```python
from build123d import *

# Parameters (mm, degrees)
SZKIC1_W                       = 168
SZKIC1_H                       = 88
ODGI_CIE_BAZOWE1_DEPTH         = 3
USKOK1_START                   = -44
USKOK1_DEPTH                   = 88
USKOK1_2_DEPTH                 = 88
SZKIC7_W                       = 60
SZKIC7_H                       = 40
WYTNIJ_WYCI_GNI_CIE1_DEPTH     = 113.751940116
ZAOKR_GLENIE1_R                = 5
OTWORY_USTALAJ_CE_6_2MM1_D     = 6.2
OTWORY_USTALAJ_CE_6_2MM1_DEPTH = 27.5
OTWORY_USTALAJ_CE_6_2MM1_TIP   = 1.862667919
OTWORY_USTALAJ_CE_8_0MM2_D     = 8.2
OTWORY_USTALAJ_CE_8_0MM2_DEPTH = 27.5
OTWORY_USTALAJ_CE_8_0MM2_TIP   = 2.463528538


# Read off the part's stored shape, not the designer's step: Uskok1
# Sheet-metal steps are written as plain solids
with BuildPart() as part:
    # Szkic1 → Odgięcie bazowe1 (new body)
    with BuildSketch(Plane(origin=(0, 0, 0), x_dir=(1, 0, 0), z_dir=(0, 1, 0))):
        Rectangle(SZKIC1_W, SZKIC1_H)
    extrude(amount=-ODGI_CIE_BAZOWE1_DEPTH)

    # Uskok1 outline → Uskok1 (cut)
    with BuildSketch(Plane.XY.offset(USKOK1_START)):
        with BuildLine():
            ThreePointArc((-10.756621532, 0), (-8.389154531, -0.845704021), (-7.093344311, -3))
            Line((-7.093344311, -3), (84, -3))
            Line((84, -3), (84, 0))
            Line((84, 0), (-10.756621532, 0))
        make_face()
    extrude(amount=USKOK1_DEPTH, mode=Mode.SUBTRACT)

    # Uskok1 2 outline → Uskok1 2 (add)
    with BuildSketch(Plane.XY.offset(USKOK1_START)):
        with BuildLine():
            ThreePointArc((-10.756621532, -3), (-10.235766677, -3.215745145), (-10.020021532, -3.7366))
            Line((-10.020021532, -3.7366), (-10.020021532, -60.2634))
            ThreePointArc((-10.020021532, -60.2634), (-8.925596731, -62.905575199), (-6.283421532, -64))
            Line((-6.283421532, -64), (84, -64))
            Line((84, -64), (84, -61))
            Line((84, -61), (-6.283421532, -61))
            ThreePointArc((-6.283421532, -61), (-6.804276387, -60.784254855), (-7.020021532, -60.2634))
            Line((-7.020021532, -60.2634), (-7.020021532, -3.7366))
            ThreePointArc((-7.020021532, -3.7366), (-7.038397411, -3.36647982), (-7.093344311, -3))
            Line((-7.093344311, -3), (-10.756621532, -3))
        make_face()
    extrude(amount=USKOK1_2_DEPTH)

    # Szkic7 → Wytnij-wyciągnięcie1 (cut, through all)
    with BuildSketch(Plane(origin=(0, -61, 0), x_dir=(1, 0, 0), z_dir=(0, 1, 0))):
        with Locations((54, 0)):
            Rectangle(SZKIC7_W, SZKIC7_H)
    extrude(amount=-WYTNIJ_WYCI_GNI_CIE1_DEPTH, mode=Mode.SUBTRACT)

    # Zaokrąglenie1
    zaokr_glenie1_edges = [part.edges().sort_by_distance(p)[0] for p in [
        (84, -62.5, -44),
        (84, -62.5, 44),
        (84, -62.5, -20),
        (84, -62.5, 20),
        (24, -62.5, 20),
        (24, -62.5, -20),
        (-84, -1.5, 44),
        (-84, -1.5, -44),
    ]]
    fillet(zaokr_glenie1_edges, radius=ZAOKR_GLENIE1_R)

    # Otwory ustalające Ø6.2mm1
    with Locations(Plane(origin=(0, -61, 0), x_dir=(1, 0, 0), z_dir=(0, 1, 0))):
        with Locations((74, 34.742873432), (74, -34.697126568), (4.56, -34.697126568), (4.56, 34.742873432)):
            Hole(OTWORY_USTALAJ_CE_6_2MM1_D / 2, depth=OTWORY_USTALAJ_CE_6_2MM1_DEPTH)
            with Locations((0, 0, -(OTWORY_USTALAJ_CE_6_2MM1_DEPTH + OTWORY_USTALAJ_CE_6_2MM1_TIP / 2))):  # 118° drill point
                Cone(0, OTWORY_USTALAJ_CE_6_2MM1_D / 2, OTWORY_USTALAJ_CE_6_2MM1_TIP, mode=Mode.SUBTRACT)

    # Otwory ustalające Ø8.0mm2
    with Locations(Plane(origin=(0, 0, 0), x_dir=(1, 0, 0), z_dir=(0, 1, 0))):
        with Locations((-69.878310766, 30), (-19.878310766, 30), (-19.878310766, -30), (-69.878310766, -30)):
            Hole(OTWORY_USTALAJ_CE_8_0MM2_D / 2, depth=OTWORY_USTALAJ_CE_8_0MM2_DEPTH)
            with Locations((0, 0, -(OTWORY_USTALAJ_CE_8_0MM2_DEPTH + OTWORY_USTALAJ_CE_8_0MM2_TIP / 2))):  # 118° drill point
                Cone(0, OTWORY_USTALAJ_CE_8_0MM2_D / 2, OTWORY_USTALAJ_CE_8_0MM2_TIP, mode=Mode.SUBTRACT)


solid = part.part
```
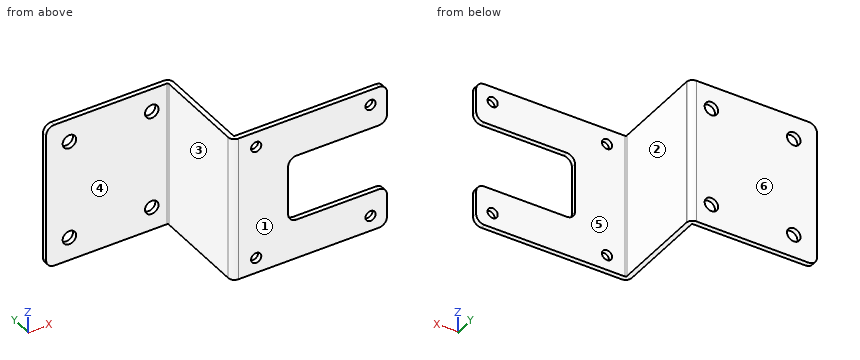
Check sheet for the modelled part. Datum: model origin and axes. Units: mm. Face numbers are marked on the shaded views. A direction names the side the tool comes from. Round coordinates to 2 decimals unless told otherwise and drop trailing zeros. Order: outer loops, then holes, each group sorted by start corner. A loop starts at its lowest first (then second) coordinate and runs counter-clockwise, first axis right, second up. Notation, with made-up numbers: (-3, 86.25) -> (2, 86.25) arc R22 ccw to (2, 98.25) -> close; hole circle Ø5 at (16, 15.25). An arc over 180 degrees is marked (long way). Use CSV: the item, a comma, the result in double quotes.
(1) Cross-section at B-B (z = -30). Record the boundary of the cut face in (x, y).
Worked out:
outline,"(-84, -3) -> (-73.98, -3) -> (-73.98, 0) -> (-84, 0) -> close; (-65.78, -3) -> (-23.98, -3) -> (-23.98, 0) -> (-65.78, 0) -> close; (-15.78, -3) -> (-10.76, -3) arc R0.74 cw to (-10.02, -3.74) -> (-10.02, -60.26) arc R3.74 ccw to (-6.28, -64) -> (84, -64) -> (84, -61) -> (-6.28, -61) arc R0.74 cw to (-7.02, -60.26) -> (-7.02, -3.74) arc R3.74 ccw to (-10.76, 0) -> (-15.78, 0) -> close"
(2) Tool access check on the marked faces 4, 5 and 6. Record the directions out of +Z, -Z, +X, -X, +Y, -Y that give a thin tool (end or side, any length) a straight path to the whole face; none if there is none.
Worked out:
face 4,"+Z, -Z, -X, -Y"
face 5,"+Z, -Z, +X, +Y"
face 6,"+Z, -Z, +X, -X, +Y"
(3) Draft check along X on the marked faces 1, 2 and 3. Enter one of: pulls with the +X half, pulls with the -X half, needs draft (parallel to the pull), parting line crosses it, or undercut.
Worked out:
face 1,"needs draft"
face 2,"pulls with the +X half"
face 3,"pulls with the -X half"
(4) Depth check by flat-ended pin: pin 1 (6.5 mm diameter, centred on x = -19.88, z = 30, fed in from +Y); pin 2 (1.5 mm diameter, centred on x = -54, z = -3, fed in from -Y); pin 3 (1 mm diameter, centred on y = -31.5, z = -9.5, fed in from -X); pin 4 (1.5 mm diameter, centred on y = -62.5, z = 7, fed in from +X). Enter the tip coordinate at first touch or a pass-through.
Worked out:
pin 1,"through"
pin 2,"y = -3"
pin 3,"x = -10.02"
pin 4,"x = 24"
(5) Cross-section at D-D (x = 49). Record the boundary of the cut face in (y, z).
Worked out:
outline,"(-64, -44) -> (-61, -44) -> (-61, -20) -> (-64, -20) -> close; (-64, 20) -> (-61, 20) -> (-61, 44) -> (-64, 44) -> close"
(6) Cross-section at A-A (x = 4.56). Record the boundary of the cut face in (y, z).
Worked out:
outline,"(-64, -44) -> (-61, -44) -> (-61, -37.84) -> (-64, -37.84) -> close; (-64, -31.64) -> (-61, -31.64) -> (-61, 31.6) -> (-64, 31.6) -> close; (-64, 37.8) -> (-61, 37.8) -> (-61, 44) -> (-64, 44) -> close"
(7) Material ranges on line 1 along Z through (x, y) = (74, -62.3); line 2 along Y through (x, z) = (41.5, -36); line 3 along X through (y, z) = (-21, 32), recorded low to high. Write a range as from..to.
Worked out:
line 1,"-44..-37.84, -31.64..-20, 20..31.6, 37.8..44"
line 2,"-64..-61"
line 3,"-10.02..-7.02"
(8) Cross-section at C-C (x = 74). Record the boundary of the cut face in (y, z).
Worked out:
outline,"(-64, -44) -> (-61, -44) -> (-61, -37.84) -> (-64, -37.84) -> close; (-64, -31.64) -> (-61, -31.64) -> (-61, -20) -> (-64, -20) -> close; (-64, 20) -> (-61, 20) -> (-61, 31.6) -> (-64, 31.6) -> close; (-64, 37.8) -> (-61, 37.8) -> (-61, 44) -> (-64, 44) -> close"
